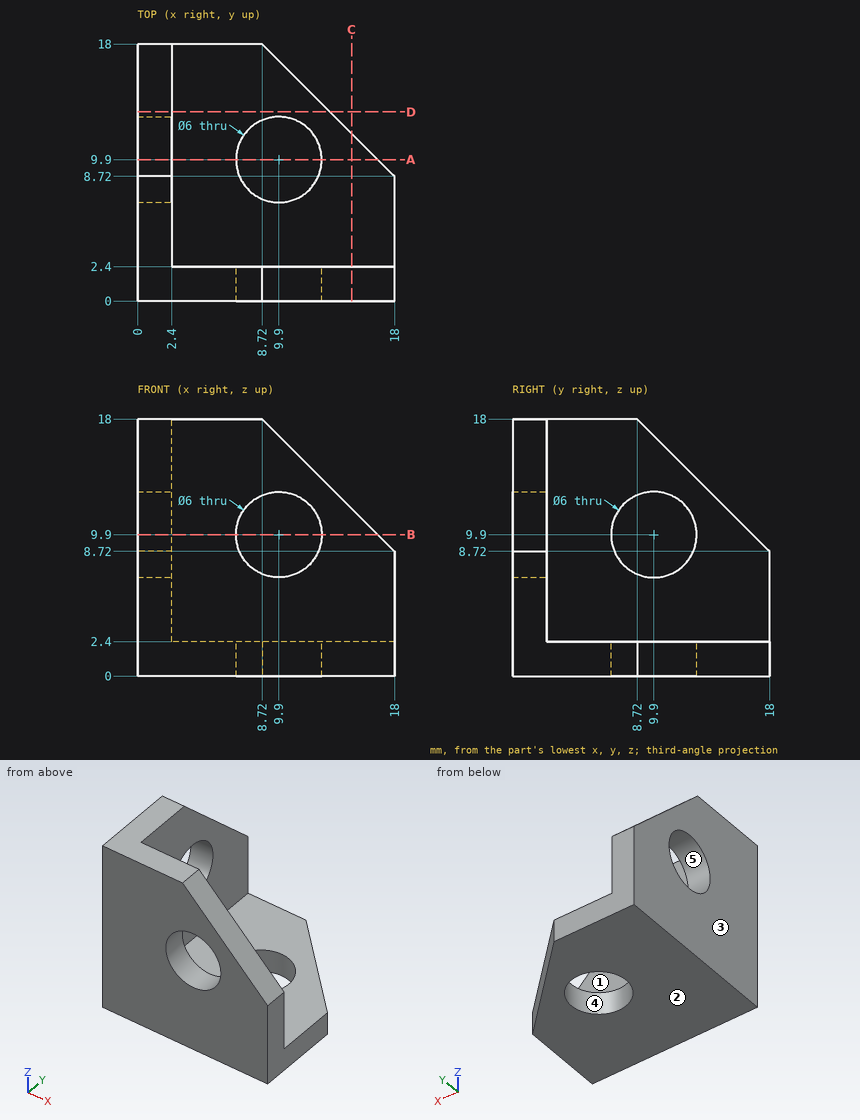
Here's the drawing with two shaded views (mm, measured from the low corner). I have some questions. A direction names the side the tool comes from. Coordinates: 2 decimals unless noted, no trailing zeros. Write each loop counter-clockwise with the first axis right and the second up, starting at its lowest first coordinate (ties: lowest second). Pieces come first, ordered by that corner, then holes.
Item 1: Will these pins go through, and if not, where does the flat tip stop? pin 1 (8 mm diameter, centred on y = 6.5, z = 12.5, fed in from +X); pin 2 (5.5 mm diameter, centred on y = 9.9, z = 9.9, fed in from +X); pin 3 (4.5 mm diameter, centred on x = 9.5, y = 8, fed in from +Z); pin 4 (4.5 mm diameter, centred on x = 9.5, z = 12, fed in from +Y).
Item 2: If I drill on line 1 (Y direction, x = 5.5, z = 17); line 2 (Y direction, x = 9, z = 2.25), over which ranges is the centre line in solid material (lowest first)?
Item 3: On a 3-axis mill with a long thin cutter (end or side, diameter ignored), from which of +Z, -Z, +X, -X, +Y, -Y can I reach the whole of each face in a straight line? I mean the marked faces 1 and 2. Say none if no direction works.
Item 4: I want a section at D-D on y = 13.25. Write out the boundary of the cut face in (x, z), and give its area (3 significant figures).
Item 5: I want a section at C-C on x = 15. Write out the boundary of the cut face in (y, z), and give its area (3 significant figures).
Item 6: I want a section at A-A on y = 9.9. Write out the boundary of the cut face in (x, z), and give its area (3 significant figures).
Item 7: If we mould it in two halves opening along X, with no side actions, what happens to the marked faces 3, 4 and 5? For each: +X half, -X half, draft (parallel to the pull), parting line (faces both ways), or undercut.
Findings below:
1. pin 1: stops at x = 2.4
1. pin 2: passes through
1. pin 3: stops at z = 2.4
1. pin 4: stops at y = 2.4
2. line 1: y = 0 to 2.4
2. line 2: y = 0 to 7.04, 12.76 to 17.72
3. face 1: +Z, +X, +Y
3. face 2: -Z, +X, -X, +Y, -Y
4. outline: (0, 0) - (13.47, 0) - (13.47, 2.4) - (2.4, 2.4) - (2.4, 13.47) - (0, 13.47) - close
4. area: 58.9 mm2
5. outline: (0, 0) - (11.72, 0) - (11.72, 2.4) - (2.4, 2.4) - (2.4, 11.72) - (0, 11.72) - close
5. area: 50.5 mm2
6. outline: (0, 0) - (6.9, 0) - (6.9, 2.4) - (2.4, 2.4) - (2.4, 6.9) - (0, 6.9) - close; (0, 12.9) - (2.4, 12.9) - (2.4, 16.82) - (0, 16.82) - close; (12.9, 0) - (16.82, 0) - (16.82, 2.4) - (12.9, 2.4) - close
6. area: 46.2 mm2
7. face 3: -X half
7. face 4: undercut
7. face 5: draft
